For this review, take the finished solid that the model builds, in its own axes (mm). Face numbers are marked on the shaded views. A direction names the side the tool comes from. Coordinates: 2 decimals unless noted, no trailing zeros. Loops run counter-clockwise (first coordinate to the right, second up) from the corner with the lowest first, then second, coordinate; pieces in that order, holes last. Notation, with made-up numbers: M 40,-11 L 60,-11 A21 ccw 60,2 Z; hole C -8.75,89.25 d4. An arc over 180 degrees is marked long. Write each question's results on one line, items separated by ' | '. Start each with the question number.
```python
from build123d import *

# Parameters (mm, degrees)
F0_W     = 50
F0_H     = 65
F1_DEPTH = 7.5
F0_W_2   = 63.5
F0_H_2   = 76.2
F2_DEPTH = 10
F3_T     = -2.5


with BuildPart() as f1:
    # F0 (on Top) → F1 (new body)
    with BuildSketch(Plane.XY):
        Rectangle(F0_W, F0_H)
    extrude(amount=F1_DEPTH)

    # F0 (on Top) → F2 (join)
    with BuildSketch(Plane.XY):
        Rectangle(F0_W_2, F0_H_2)
        Rectangle(F0_W, F0_H, mode=Mode.SUBTRACT)
    extrude(amount=F2_DEPTH)

    # F3
    f3_openings = [f1.faces().sort_by_distance(p)[0] for p in [
        (0, 0, 0),
    ]]
    offset(amount=F3_T, openings=f3_openings, kind=Kind.INTERSECTION)


solid = f1.part
```
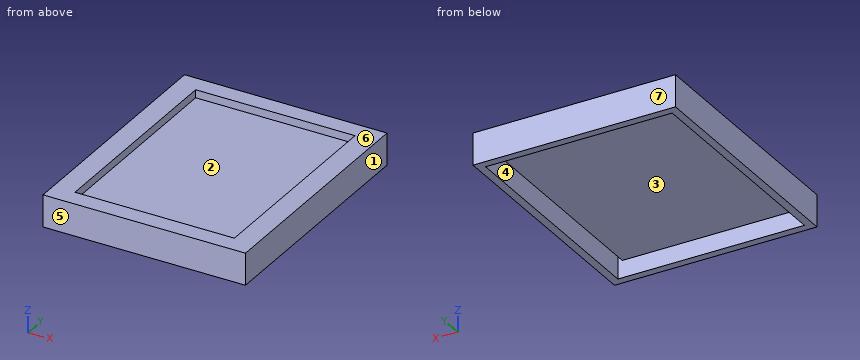
Q1. For the marked faces 1, 2 and 3, list the 3-axis set-ups (+Z, -Z, +X, -X, +Y, -Y) from which the entire face can be reached by the end or side of a thin tool; tool diameter is ignored.
Q2. Insertion check: P1, Ø2, axis at x = 14, y = 24, coming from the +Z side. The pin has a flat end and moves straight along its axis. Give the tip position at first contact, or say it passes through.
Q3. Take a section at A-A, the plane z = 9. Give the boundary of the cut face in (x, y).
Q4. Take a section at D-D, the plane z = 3.75. Give the boundary of the cut face in (x, y).
Q5. The part is to be moulded in two halves that separate along Y. For the marked faces 4, 5, 6 and 7, say which applies: pulls with the +Y half, pulls with the -Y half, needs draft (parallel to the pull), parting line crosses it, or undercut.
Q6. Take a section at C-C, the plane x = 26.5. Give the boundary of the cut face in (y, z), then the cut area to 3 significant figures.
Q7. Take a section at B-B, the plane y = 13.5. Give the boundary of the cut face in (x, z).
Q8. To check wall thickness, follow line 1 along X through (y, z) = (-4, 2.75); line 2 along Y through (x, z) = (-17, 8.75); line 3 along X through (y, z) = (25, 5.25). State the ranges of each line that lie inside material, in increasing order.
Results:
1) face 1: +Z, -Z, +X, +Y, -Y | face 2: +Z | face 3: -Z
2) P1: z = 7.5
3) outline: M -31.75,-38.1 L 31.75,-38.1 L 31.75,38.1 L -31.75,38.1 Z; hole M -25,-32.5 L 25,-32.5 L 25,32.5 L -25,32.5 Z
4) outline: M -31.75,-38.1 L 31.75,-38.1 L 31.75,38.1 L -31.75,38.1 Z; hole M -29.25,-35.6 L 29.25,-35.6 L 29.25,35.6 L -29.25,35.6 Z
5) face 4: undercut | face 5: pulls with the -Y half | face 6: needs draft | face 7: pulls with the +Y half
6) outline: M -38.1,0 L -35.6,0 L -35.6,7.5 L -35,7.5 L -35,5 L 35,5 L 35,7.5 L 35.6,7.5 L 35.6,0 L 38.1,0 L 38.1,10 L -38.1,10 Z | area: 403 mm^2
7) outline: M -31.75,0 L -29.25,0 L -29.25,7.5 L -27.5,7.5 L -27.5,5 L 27.5,5 L 27.5,7.5 L 29.25,7.5 L 29.25,0 L 31.75,0 L 31.75,10 L 25,10 L 25,7.5 L -25,7.5 L -25,10 L -31.75,10 Z
8) line 1: -31.75 to -29.25, 29.25 to 31.75 | line 2: -38.1 to -32.5, 32.5 to 38.1 | line 3: -31.75 to -29.25, -27.5 to 27.5, 29.25 to 31.75
